```python
from build123d import *

# Parameters (mm, degrees)
BOSS_EXTRUDE1_DEPTH = 3.5
SKETCH2_R           = 1.375
CUT_EXTRUDE1_DEPTH  = 47.767592889
BOSS_EXTRUDE5_DEPTH = 6
SKETCH9_R           = 1
CUT_EXTRUDE2_DEPTH  = 10


with BuildPart() as part:
    # Sketch1 → Boss-Extrude1 (new body)
    with BuildSketch(Plane(origin=(0, 0, 0), x_dir=(1, 0, 0), z_dir=(0, 1, 0))):
        with BuildLine():
            Line((5.65, -1.875), (5.65, 1.875))
            Line((5.65, 1.875), (1.9, 1.875))
            Line((1.9, 1.875), (-1.875, -31))
            Line((-1.875, -31), (-17.265, -31))
            Line((-17.265, -31), (-21.04, 1.875))
            Line((-21.04, 1.875), (-24.79, 1.875))
            Line((-24.79, 1.875), (-24.79, -1.875))
            Line((-24.79, -1.875), (-23.673675208, -11.929569188))
            ThreePointArc((-23.673675208, -11.929569188), (-25.440763963, -14.138052226), (-23.232280925, -15.905140982))
            Line((-23.232280925, -15.905140982), (-21.14, -34.75))
            Line((-21.14, -34.75), (-19.14, -34.75))
            Line((-19.14, -34.75), (0, -34.75))
            Line((0, -34.75), (2, -34.75))
            Line((2, -34.75), (4.092280925, -15.905140982))
            ThreePointArc((4.092280925, -15.905140982), (6.300763963, -14.138052226), (4.533675208, -11.929569188))
            Line((4.533675208, -11.929569188), (5.65, -1.875))
        make_face()
    boss_extrude1 = extrude(amount=BOSS_EXTRUDE1_DEPTH)

    # Sketch2 → Cut-Extrude1 (cut, through all)
    with BuildSketch(Plane(origin=(5.65, 0, 0), x_dir=(0, 0, -1), z_dir=(1, 0, 0))):
        with Locations((0, 1.75)):
            Circle(SKETCH2_R)
    cut_extrude1 = extrude(amount=-CUT_EXTRUDE1_DEPTH, mode=Mode.SUBTRACT)

    # Sketch7 → Boss-Extrude5 (add)
    with BuildSketch(Plane(origin=(0, 3.5, 0), x_dir=(1, 0, 0), z_dir=(0, 1, 0))):
        Polygon((-1.875, -31), (-1.875, -34.75), (2, -34.75), (2.41634981, -31), align=None)
        Polygon((-21.55634981, -31), (-17.265, -31), (-17.265, -34.75), (-21.14, -34.75), align=None)
    boss_extrude5 = extrude(amount=BOSS_EXTRUDE5_DEPTH)

    # Mirror46: Boss-Extrude1, Cut-Extrude1, Boss-Extrude5 across plane
    add(boss_extrude1.mirror(Plane.XY))
    add(cut_extrude1.mirror(Plane.XY), mode=Mode.SUBTRACT)
    add(boss_extrude5.mirror(Plane.XY))

    # Sketch9 → Cut-Extrude2 (cut)
    with BuildSketch(Plane(origin=(0, 3.5, 0), x_dir=(1, 0, 0), z_dir=(0, 1, 0))):
        with Locations(Location((4.28, 13.85, 0), (0, 0, 270))):
            Circle(SKETCH9_R)
        with Locations(Location((-23.42, 13.85, 0), (0, 0, 270))):
            Circle(SKETCH9_R)
        with Locations(Location((-23.42, -13.85, 0), (0, 0, 270))):
            Circle(SKETCH9_R)
        with Locations(Location((4.28, -13.85, 0), (0, 0, 270))):
            Circle(SKETCH9_R)
    extrude(amount=-CUT_EXTRUDE2_DEPTH, mode=Mode.SUBTRACT)


solid = part.part
```
The listing builds one solid part. Answer for the finished solid, in the listing's coordinates (mm). A direction names the side the tool comes from. Round coordinates to 2 decimals unless told otherwise and drop trailing zeros. Write each loop counter-clockwise with the first axis right and the second up, starting at its lowest first coordinate (ties: lowest second). Pieces come first, ordered by that corner, then holes. Notation, with made-up numbers: (56, -21.5) -> (67, -21.5) arc R24 cw to (67, -0.5) -> close; hole circle Ø6 at (31.5, -33). An arc over 180 degrees is marked (long way). Write item = value, one per line.
1) Section B-B on x = -5 is taken. Write down the section's boundary in (y, z), plus the area to 4 significant figures.
Check values:
outline = (0, -34.75) -> (3.5, -34.75) -> (3.5, -31) -> (0, -31) -> close; (0, 31) -> (3.5, 31) -> (3.5, 34.75) -> (0, 34.75) -> close
area = 26.25 mm²
2) Section D-D on z = -13.5 is taken. Write down the section's boundary in (x, y).
Check values:
outline = (-25.41, 0) -> (-24.36, 0) -> (-24.36, 3.5) -> (-25.41, 3.5) -> close; (-22.48, 0) -> (-19.27, 0) -> (-19.27, 3.5) -> (-22.48, 3.5) -> close; (0.13, 0) -> (3.34, 0) -> (3.34, 3.5) -> (0.13, 3.5) -> close; (5.22, 0) -> (6.27, 0) -> (6.27, 3.5) -> (5.22, 3.5) -> close
3) Section A-A on y = 8.5 is taken. Write down the section's boundary in (x, z) (3 decimals), plus the area to 3 significant figures.
Check values:
outline = (-21.556, -31) -> (-21.14, -34.75) -> (-17.265, -34.75) -> (-17.265, -31) -> close; (-21.556, 31) -> (-17.265, 31) -> (-17.265, 34.75) -> (-21.14, 34.75) -> close; (-1.875, -34.75) -> (2, -34.75) -> (2.416, -31) -> (-1.875, -31) -> close; (-1.875, 31) -> (2.416, 31) -> (2, 34.75) -> (-1.875, 34.75) -> close
area = 61.2 mm²
4) Section C-C on y = 2.5 is taken. Give the number of separate pieces and of enclosed holes in the cut face, plus the area to 3 significant figures.
Check values:
separate_pieces = 2
enclosed_holes = 4
area = 695 mm²
5) Which of the six approach directions +Z, -Z, +X, -X, +Y, -Y give full straight-line access (tool end or side, diameter ignored) to faces 4 (the flat face through (-0.07, 1.73, -15.28)), 5 (the flat face through (2, 3.5, 0)), 6 (the flat face through (5.084, 1.726, -6.973)), 7 (the flat face through (-17.265, 6, -33)), 8 (the flat face through (-24.24, 1.73, 6.83))?
Check values:
face_4 = +Y, -Y
face_5 = +X, -X, +Y
face_6 = +X, +Y, -Y
face_7 = +Z, -Z, +Y
face_8 = -X, +Y, -Y
6) Given pin 1 (4 mm diameter, centred on x = -7.5, z = -32, fed in from +Y); pin 2 (1.9 mm diameter, centred on y = 5, z = -32, fed in from -X); pin 3 (1.1 mm diameter, centred on y = 5, z = -33, fed in from +X); pin 4 (3 mm diameter, centred on x = -2, y = 7, fed in from -Z), each flat-ended and moving along its own axis, determine where each tip first touches the part or whether it passes through.
Check values:
pin_1 = 3.5
pin_2 = -21.55
pin_3 = 2.26
pin_4 = -34.75
7) For a pull along X with two mould halves and no side action, classify faces 1 (the flat face through (-19.02, 1.73, -15.72)), 2 (the flat face through (-19, 6, -31)), 3 (the flat face through (-24.24, 1.73, -6.83)) as released by +X, released by -X, zero draft, split by the parting line, or undercut.
Check values:
face_1 = undercut
face_2 = zero draft
face_3 = released by -X
8) Straight lines are drawn through the part: line 1 along X through (y, z) = (2.8, 13.85); line 2 along Y through (x, z) = (2.4, 0) (3 decimals); line 3 along Z through (x, y) = (-21, 6.5). For each, find the intervals that lie inside material, in ascending order. Write a range as [from, to].
Check values:
line_1 = [-25.45, -24.42], [-22.42, -19.23], [0.09, 3.28], [5.28, 6.31]
line_2 = [0, 0.375], [3.125, 3.5]
line_3 = [-34.75, -31], [31, 34.75]
